Read the model definition and answer for the solid it produces. Units are mm, in the model's axes. A direction names the side the tool comes from. Give positions to 0.01 mm unless a question says otherwise; leave off trailing zeros. Order: outer loops, then holes, each group sorted by start corner. A loop starts at its lowest first (then second) coordinate and runs counter-clockwise, first axis right, second up. Notation, with made-up numbers: (1, 14) - (54, 14) arc R16 ccw to (54, 27) - close; hole circle Ø10 at (-19, 66). An arc over 180 degrees is marked (long way). One line per item, written item: value. Start each with the question number.
```python
from build123d import *

# Parameters (mm, degrees)
SKETCH1_R            = 3.5
BOSS_EXTRUDE2_DEPTH  = 8.75
BOSS_EXTRUDE3_DEPTH  = 6.5
SKETCH2_R            = 5
BOSS_EXTRUDE4_DEPTH  = 0.5
SKETCH4_W            = 6
SKETCH4_H            = 8.25
BOSS_EXTRUDE5_DEPTH  = 6
SKETCH5_W            = 0.5
SKETCH5_H            = 0.45
CUT_EXTRUDE2_DEPTH   = 13.57477634
LPATTERN1_COUNT      = 4
LPATTERN1_PITCH      = 0.9
LPATTERN1_COUNT_DIR2 = 2
LPATTERN1_PITCH_DIR2 = 5.5
SKETCH6_R            = 3
SKETCH6_R_2          = 0.75
CUT_EXTRUDE3_DEPTH   = 8.75
SKETCH7_R            = 0.75
CUT_EXTRUDE4_DEPTH   = 13.927683474
SKETCH8_R            = 0.375
CUT_EXTRUDE5_DEPTH   = 0.5


with BuildPart() as part:
    # Sketch1 → Boss-Extrude2 (new body)
    with BuildSketch(Plane(origin=(0, 0, 0), x_dir=(1, 0, 0), z_dir=(0, 1, 0))):
        with Locations(Location((0, 0, 0), (0, 0, 270))):
            Circle(SKETCH1_R)
    extrude(amount=BOSS_EXTRUDE2_DEPTH)

    # Sketch1_3 → Boss-Extrude3 (add)
    with BuildSketch(Plane(origin=(0, 0, 0), x_dir=(1, 0, 0), z_dir=(0, 1, 0))):
        with BuildLine():
            Line((-3.312648335, 1.129761483), (-6, -6.75))
            Line((-6, -6.75), (6, -6.75))
            Line((6, -6.75), (3.312648335, 1.129761483))
            ThreePointArc((3.312648335, 1.129761483), (3.45284442, 0.572595332), (3.5, 0))
            ThreePointArc((3.5, 0), (-0.572595332, -3.45284442), (-3.312648335, 1.129761483))
        make_face()
    extrude(amount=BOSS_EXTRUDE3_DEPTH)

    # Sketch2 → Boss-Extrude4 (add)
    with BuildSketch(Plane(origin=(0, 8.75, 0), x_dir=(1, 0, 0), z_dir=(0, 1, 0))):
        with Locations(Location((0, 0, 0), (0, 0, 270))):
            Circle(SKETCH2_R)
    extrude(amount=BOSS_EXTRUDE4_DEPTH)

    # Sketch4 → Boss-Extrude5 (add)
    with BuildSketch(Plane.XY.offset(-6)):
        with Locations((0, 4.625)):
            Rectangle(SKETCH4_W, SKETCH4_H)
    extrude(amount=BOSS_EXTRUDE5_DEPTH)

    # Sketch5 → Cut-Extrude2 (cut, through all)
    with BuildSketch(Plane(origin=(0, 8.75, 0), x_dir=(1, 0, 0), z_dir=(0, 1, 0))):
        with Locations((2.75, 5.325)):
            Rectangle(SKETCH5_W, SKETCH5_H)
    cut_extrude2 = extrude(amount=-CUT_EXTRUDE2_DEPTH, mode=Mode.SUBTRACT)

    # LPattern1: Cut-Extrude2 4 × 2
    with Locations(*[(-j * LPATTERN1_PITCH_DIR2, 0, i * LPATTERN1_PITCH) for i in range(LPATTERN1_COUNT) for j in range(LPATTERN1_COUNT_DIR2) if (i, j) != (0, 0)]):
        add(cut_extrude2, mode=Mode.SUBTRACT)

    # Sketch6 → Cut-Extrude3 (cut)
    with BuildSketch(Plane(origin=(0, 9.25, 0), x_dir=(1, 0, 0), z_dir=(0, 1, 0))):
        with Locations(Location((0, 0, 0), (0, 0, 270))):
            Circle(SKETCH6_R)
        with Locations(Location((0, 0, 0), (0, 0, 270))):
            Circle(SKETCH6_R_2, mode=Mode.SUBTRACT)
    extrude(amount=-CUT_EXTRUDE3_DEPTH, mode=Mode.SUBTRACT)

    # Sketch7 → Cut-Extrude4 (cut, through all)
    with BuildSketch(Plane(origin=(0, 9.25, 0), x_dir=(1, 0, 0), z_dir=(0, 1, 0))):
        with Locations(Location((0, 0, 0), (0, 0, 270))):
            Circle(SKETCH7_R)
    extrude(amount=-CUT_EXTRUDE4_DEPTH, mode=Mode.SUBTRACT)

    # Sketch8 → Cut-Extrude5 (cut)
    with BuildSketch(Plane(origin=(0, 9.25, 0), x_dir=(1, 0, 0), z_dir=(0, 1, 0))):
        with Locations(Location((0, -4.25, 0), (0, 0, 270))):
            Circle(SKETCH8_R)
        with Locations(Location((-3.680607966, 2.125, 0), (0, 0, 270))):
            Circle(SKETCH8_R)
        with Locations(Location((3.680607966, 2.125, 0), (0, 0, 270))):
            Circle(SKETCH8_R)
    extrude(amount=-CUT_EXTRUDE5_DEPTH, mode=Mode.SUBTRACT)


solid = part.part
```
1) Find the intervals of material crossed by probe 1 along Y at (x, z) = (-1.5, 4); probe 2 along X at (y, z) = (0.3, 0); probe 3 along Y at (x, z) = (-2, 1.5), in increasing order. Write a range as from..to.
2) The mould has two halves that part along X. Classify faces 4 (the cylindrical face through (0.225, 0.254, 0.715)), 5 (the flat face through (-3.3, 9.25, -0.1)), 6 (the flat face through (-1, 0.5, 1)), 7 (the flat face through (-4.638, 3.204, 2.755)): +X half, -X half, draft (parallel to the pull), parting line (faces both ways), or undercut.
3) Section A-A on x = 0 is taken. Write down the section's boundary in (y, z) (3 decimals).
4) Section D-D on z = 2.25 is taken. Write down the section's boundary in (x, y).
5) Each of these flat-tipped pins is pushed along its axis until it touches: pin 1 (0.5 mm diameter, centred on y = 6, z = -3, fed in from -X); pin 2 (0.5 mm diameter, centred on y = 5, z = -4.5, fed in from +X); pin 3 (1.5 mm diameter, centred on y = 6.5, z = -1, fed in from -X). Where does it stop, or does it pass through?
6) Section C-C on z = 4.25 is taken. Write down the section's boundary in (x, y) (3 decimals).
7) Section B-B on z = 0 is taken. Write down the section's boundary in (x, y).
8) For faces 1 (the cylindrical face through (0, 0.2, -3.5)), 2 (the flat face through (0, 8.75, -5.4)), 3 (the cylindrical face through (0.9, 4.94, 2.86)), determine the directions among +Z, -Z, +X, -X, +Y, -Y from which every point of the face is accessible in a straight line to the end or side of a thin tool.
Solved:
1. probe 1: y = 0..6.5, 8.75..9.25
1. probe 2: x = -3.7..-0.75, 0.75..3.7
1. probe 3: y = 0..0.5
2. face 4: undercut
2. face 5: draft
2. face 6: undercut
2. face 7: -X half
3. outline: (0, -3.5) - (0.5, -3.5) - (0.5, -6) - (8.75, -6) - (8.75, -5) - (9.25, -5) - (9.25, -3) - (0.5, -3) - (0.5, -0.75) - (0, -0.75) - close; (0, 0.75) - (0.5, 0.75) - (0.5, 3) - (9.25, 3) - (9.25, 3.875) - (8.75, 3.875) - (8.75, 3.5) - (6.5, 3.5) - (6.5, 6.75) - (0, 6.75) - close; (8.75, 4.625) - (9.25, 4.625) - (9.25, 5) - (8.75, 5) - close
4. outline: (-4.47, 0) - (4.47, 0) - (4.47, 6.5) - (2.68, 6.5) - (2.68, 8.75) - (4.47, 8.75) - (4.47, 9.25) - (1.98, 9.25) - (1.98, 0.5) - (-1.98, 0.5) - (-1.98, 9.25) - (-4.47, 9.25) - (-4.47, 8.75) - (-2.68, 8.75) - (-2.68, 6.5) - (-4.47, 6.5) - close
5. pin 1: stops at x = -3
5. pin 2: stops at x = 3
5. pin 3: stops at x = -3.61
6. outline: (-5.147, 0) - (5.147, 0) - (5.147, 6.5) - (-5.147, 6.5) - close; (-2.634, 8.75) - (-0.375, 8.75) - (-0.375, 9.25) - (-2.634, 9.25) - close; (0.375, 8.75) - (2.634, 8.75) - (2.634, 9.25) - (0.375, 9.25) - close
7. outline: (-5, 8.75) - (-3.5, 8.75) - (-3.5, 6.5) - (-3.7, 6.5) - (-3.7, 0) - (-0.75, 0) - (-0.75, 0.5) - (-3, 0.5) - (-3, 9.25) - (-5, 9.25) - close; (0.75, 0) - (3.7, 0) - (3.7, 6.5) - (3.5, 6.5) - (3.5, 8.75) - (5, 8.75) - (5, 9.25) - (3, 9.25) - (3, 0.5) - (0.75, 0.5) - close
8. face 1: -Z, -Y
8. face 2: -Z, +Y
8. face 3: +Y
